Verification items for the finished model (mm, model axes). Face numbers are marked on the shaded views. A direction names the side the tool comes from. Coordinates: 2 decimals unless noted, no trailing zeros. Write each loop counter-clockwise with the first axis right and the second up, starting at its lowest first coordinate (ties: lowest second). Pieces come first, ordered by that corner, then holes. Notation, with made-up numbers: (-34.75, 65.25) - (19.25, 65.25) arc R28 ccw to (19.25, 93.25) - close; hole circle Ø9 at (1, 10). An arc over 180 degrees is marked (long way). Use CSV: the item, a comma, the result in double quotes. Start each with the question number.
Autodesk Inventor part; units mm, degrees
ref_plane "YZ Plane" through (0, 0, 0) normal (1, 0, 0) x (0, 1, 0)
ref_plane "XZ Plane" through (0, 0, 0) normal (0, 1, 0) x (-1, 0, 0)
ref_plane "XY Plane" through (0, 0, 0) normal (0, 0, 1) x (1, 0, 0)
sketch "Sketch1" plane through (0, 0, 0) normal (0, 1, 0) x (-1, 0, 0)
  line L0 (11, 20) -> (-11, 20)
  line L1 (-11, 20) -> (-11, -20)
  line L2 (-11, -20) -> (11, -20)
  line L3 (11, -20) -> (11, 20)
  line L4 (11, 20) -> (-11, -20) construction
  line L5 (-11, 20) -> (11, -20) construction
  dimension "d0" = 22
  dimension "d1" = 40
extrude "Extrusion1" add sketch "Sketch1" along normal blind 15
sketch "Sketch2" plane through (0, 15, 0) normal (0, 1, 0) x (1, 0, 0)
  line L0 (-8, -17) -> (8, -17)
  line L1 (8, -17) -> (8, 17)
  line L2 (8, 17) -> (-8, 17)
  line L3 (-8, 17) -> (-8, -17)
  line L4 (-8, -17) -> (8, 17) construction
  line L5 (8, -17) -> (-8, 17) construction
  point P0 (0, 0)
  dimension "d6" = 16
  dimension "d7" = 34
extrude "Extrusion2" cut sketch "Sketch2" against normal blind 3
sketch "Sketch3" plane through (0, 12, 0) normal (0, 1, 0) x (1, 0, 0)
  line L0 (6, -17) -> (-6, -17)
  line L1 (-6, -17) -> (-6, 17)
  line L2 (-6, 17) -> (6, 17)
  line L3 (6, 17) -> (6, -17)
  line L4 (6, -17) -> (-6, 17) construction
  line L5 (-6, -17) -> (6, 17) construction
  point P0 (0, 0)
  dimension "d10" = 12
  dimension "d11" = 34
extrude "Extrusion3" cut sketch "Sketch3" against normal blind 3
sketch "Sketch4" plane through (0, 15, 0) normal (0, 1, 0) x (1, 0, 0)
  line L0 (-7, 9) -> (7, 9)
  line L1 (7, 9) -> (7, 17)
  line L2 (7, 17) -> (-7, 17)
  line L3 (-7, 17) -> (-7, 9)
  line L4 (-7, 9) -> (7, 17) construction
  line L5 (7, 9) -> (-7, 17) construction
  point P0 (0, 0)
  point P1 (0, 13)
  dimension "d14" = 14
  dimension "d15" = 8
extrude "Extrusion4" cut sketch "Sketch4" against normal through all
sketch "Sketch5" plane through (0, 9, 0) normal (0, 1, 0) x (1, 0, 0)
  circle A0 centre (0, -9) radius 3
  point P0 (0, 0)
  dimension "d18" = 6
extrude "Extrusion5" add sketch "Sketch5" along normal up to surface (3 mm away)
sketch "Sketch6" plane through (0, 12, 9) normal (0, 1, 0) x (1, 0, 0)
  point P0 (0, 9)
  point P1 (0, 0)
  point P2 (0, 0)
hole "Hole1" at (0, 12, 9) direction (0, -1, 0) diameter 3.6 end through all
sketch "Sketch7" plane through (0, 0, 0) normal (0, -1, 0) x (1, 0, 0)
  circle A0 centre (0, 9) radius 1.8
  line L0 (1.7032, 11.95) -> (3.4064, 9)
  line L1 (3.4064, 9) -> (1.7032, 6.05)
  line L2 (1.7032, 6.05) -> (-1.7032, 6.05)
  line L3 (-1.7032, 6.05) -> (-3.4064, 9)
  line L4 (-3.4064, 9) -> (-1.7032, 11.95)
  line L5 (-1.7032, 11.95) -> (1.7032, 11.95)
  point P0 (0, 0)
  point P1 (0, 11.95)
extrude "Extrusion6" cut sketch "Sketch7" against normal blind 5
properties part number "Holder"
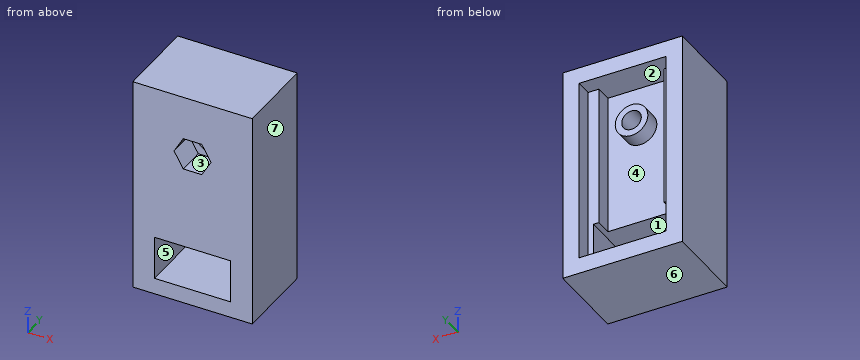
Q1. Cross-section at B-B (y = 4.25). Record the cut outline in (x, z), plus the area to 3 significant figures.
Q2. Cross-section at D-D (z = -14). Record the cut outline in (x, y).
Q3. Scan lines: line 1 along Z through (x, y) = (0, 8.25); line 2 along Z through (x, y) = (1.5, 13.5); line 3 along X through (y, z) = (5.25, -16.5). Record each from-to range of solid material in increasing order. Write a range as from..to.
Q4. Release check for a two-part mould opening along Z. For the marked faces 4, 5, 6 and 7 record: released by +Z, released by -Z, zero draft, split by the parting line, or undercut.
Q5. Gauge pin test, flat ends, axial feed: pin 1 (0.6 mm diameter, centred on x = -7.5, z = -6, fed in from +Y); pin 2 (3 mm diameter, centred on x = 0, z = -2.5, fed in from +Y); pin 3 (3 mm diameter, centred on x = 0, z = 9, fed in from -Y). Record the tip position at first contact, or that the pin passes through.
Q6. Tool access check on the marked faces 1, 2 and 3. Record the directions out of +Z, -Z, +X, -X, +Y, -Y that give a thin tool (end or side, any length) a straight path to the whole face; none if there is none.
Q7. Cross-section at A-A (x = 0). Record the cut outline in (y, z).
Q8. Cross-section at C-C (x = 4.75). Record the cut outline in (y, z).
Reply:
1,outline,"(-11, -20) - (11, -20) - (11, 20) - (-11, 20) - close; hole (-7, -17) - (7, -17) - (7, -9) - (-7, -9) - close; hole (-3.41, 9) - (-1.7, 6.05) - (1.7, 6.05) - (3.41, 9) - (1.7, 11.95) - (-1.7, 11.95) - close"
1,area,"738 mm^2"
2,outline,"(-11, 0) - (-7, 0) - (-7, 12) - (-8, 12) - (-8, 15) - (-11, 15) - close; (7, 0) - (11, 0) - (11, 15) - (8, 15) - (8, 12) - (7, 12) - close"
3,line 1,"-20..-17, -9..7.2, 10.8..20"
3,line 2,"-20..-17, 17..20"
3,line 3,"-11..-7, 7..11"
4,face 4,"undercut"
4,face 5,"undercut"
4,face 6,"released by -Z"
4,face 7,"zero draft"
5,pin 1,"y = 12"
5,pin 2,"y = 9"
5,pin 3,"through"
6,face 1,"+Y, -Y"
6,face 2,"+Y"
6,face 3,"-Y"
7,outline,"(0, -20) - (15, -20) - (15, -17) - (0, -17) - close; (0, -9) - (9, -9) - (9, 6) - (12, 6) - (12, 7.2) - (5, 7.2) - (5, 6.05) - (0, 6.05) - close; (0, 11.95) - (5, 11.95) - (5, 10.8) - (12, 10.8) - (12, 12) - (9, 12) - (9, 17) - (15, 17) - (15, 20) - (0, 20) - close"
8,outline,"(0, -20) - (15, -20) - (15, -17) - (0, -17) - close; (0, -9) - (9, -9) - (9, 17) - (15, 17) - (15, 20) - (0, 20) - close"
